Part print with two shaded views. Sizes in mm from the minimum x, y, z corner. A direction names the side the tool comes from. Round coordinates to 2 decimals unless told otherwise and drop trailing zeros. Write each loop counter-clockwise with the first axis right and the second up, starting at its lowest first coordinate (ties: lowest second). Pieces come first, ordered by that corner, then holes. Notation, with made-up numbers: M 24,-31.5 L 71,-31.5 A27 cw 71,-8.5 Z; hole C 15,48 d4. An arc over 180 degrees is marked long. Use one line per item in the form item = value. Start each with the question number.
Item 1: Which spindle directions (+Z, -Z, +X, -X, +Y, -Y) get a long thin tool onto all of the face, cutting with end or side? Do the marked faces 1 and 2. Say none if no direction does.
Item 2: Cut at C-C, the plane z = 0.6. Give the cut face in (x, y).
Item 3: Cut at B-B, the plane y = 0.4. Give the cut face in (x, z).
Item 4: Probe L1, parallel to X at y = 2.45, z = 1.8; L2, parallel to X at y = 3.05, z = 2.9; L3, parallel to Y at x = 6.25, z = 3.15. List the from-to ranges inside material, lowest first.
Item 5: Flat gauge pin, fed straight in: pin 1 Ø1.8 at (x, z) = (7.5, 2) entering from +Y. Where does the tip first touch, or does it go through?
Item 6: Cut at A-A, the plane y = 2.85. Give the cut face in (x, z), then the cut area to 3 significant figures.
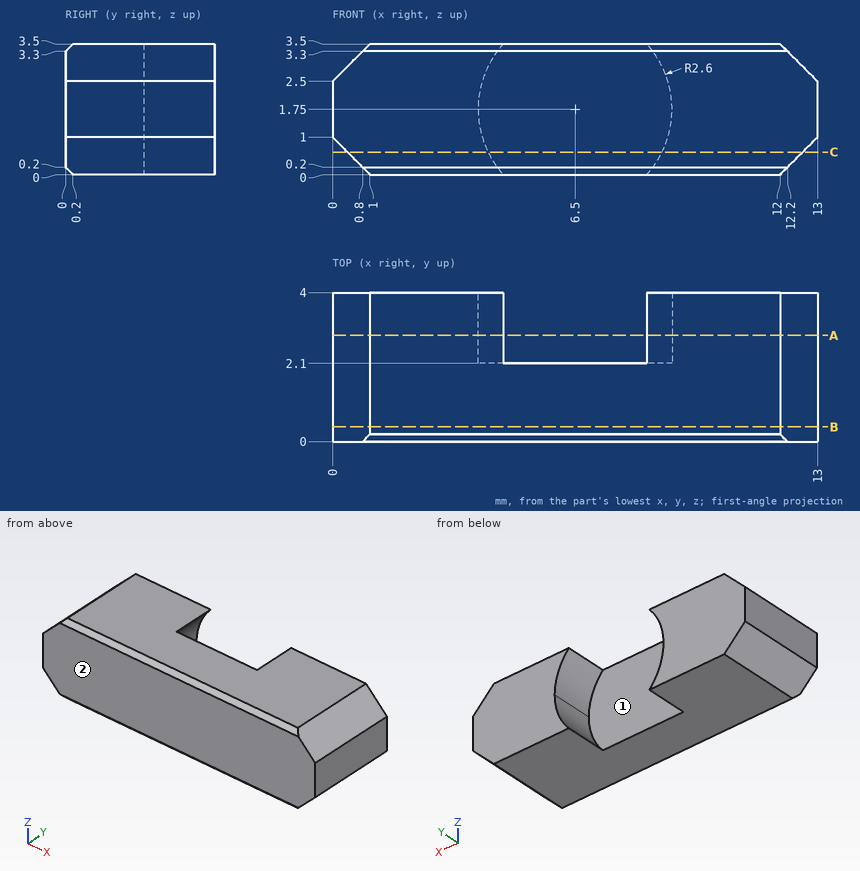
Model answer:
q1.face_1 = +Y
q1.face_2 = +Z, -Z, +X, -X, -Y
q2.outline = M 0.4,0 L 12.6,0 L 12.6,4 L 8.83,4 L 8.83,2.1 L 4.17,2.1 L 4.17,4 L 0.4,4 Z
q3.outline = M 0,1 L 1,0 L 12,0 L 13,1 L 13,2.5 L 12,3.5 L 1,3.5 L 0,2.5 Z
q4.L1 = 0 to 3.9, 9.1 to 13
q4.L2 = 0.4 to 4.17, 8.83 to 12.6
q4.L3 = 0 to 2.1
q5.pin_1 = 2.1
q6.outline = M 0,1 L 1,0 L 4.58,0 A2.6 cw 4.58,3.5 L 1,3.5 L 0,2.5 Z; M 8.42,0 L 12,0 L 13,1 L 13,2.5 L 12,3.5 L 8.42,3.5 A2.6 cw Z
q6.area = 26.8 mm²
